from build123d import *

# Parameters (mm, degrees)
SKETCH_R   = 14.3256
SKETCH_R_2 = 38.1
PAD_DEPTH  = 10.000005


with BuildPart() as part:
    # Sketch → Pad (new body)
    with BuildSketch(Plane.XY):
        with BuildLine():
            Line((0, 304.8), (0, 0))
            Line((0, 0), (-203.3016, 0))
            Line((-203.3016, 0), (-203.3016, 304.8))
            ThreePointArc((0, 304.8), (-101.6508, 400.298945), (-203.3016, 304.8))
        make_face()
        with Locations((-152.4, 50.9016)):
            Circle(SKETCH_R, mode=Mode.SUBTRACT)
        with Locations((-50.9016, 50.9016)):
            Circle(SKETCH_R, mode=Mode.SUBTRACT)
        with Locations((-152.4, 152.4)):
            Circle(SKETCH_R, mode=Mode.SUBTRACT)
        with Locations((-50.8, 152.4)):
            Circle(SKETCH_R, mode=Mode.SUBTRACT)
        with Locations((-152.4, 254)):
            Circle(SKETCH_R, mode=Mode.SUBTRACT)
        with Locations((-50.8, 254)):
            Circle(SKETCH_R, mode=Mode.SUBTRACT)
        with Locations((-101.6, 304.8)):
            Circle(SKETCH_R_2, mode=Mode.SUBTRACT)
    extrude(amount=PAD_DEPTH)


solid = part.part
Geometry: final body of the model. Coordinates: model frame, mm. Give positions to 0.01 mm unless a question says otherwise; leave off trailing zeros. Loops run counter-clockwise (first coordinate to the right, second up) from the corner with the lowest first, then second, coordinate; pieces in that order, holes last. Notation, with made-up numbers: (4, 45) - (14, 45) arc R5 cw to (14, 51) - close; hole circle Ø6 at (-25, 34). An arc over 180 degrees is marked (long way). One line per question, with ' | ' between items. Start each with the question number.
(1) Section query C-C on z = 1.75. Return loops of the section in (x, y).
(2) Ray query, line 1 (X direction, y = 253, z = 6); line 2 (Y direction, x = -50.8, z = 3.25); line 3 (Y direction, x = -57.5, z = 4). Return the intervals inside material, ascending. Write a range as from..to.
(3) Pull-direction query (X, two-part tool) for faces 1 (the cylindrical face through (-53.906, 240.015, 4.93)), 2 (the flat face through (-203.302, 150, 5)), 3 (the flat face through (-100, 0, 5)), 4 (the cylindrical face through (-84.02, 271, 4.93)); classes: released by +X, released by -X, zero draft, split by the parting line, or undercut.
(4) Section query A-A on y = 254. Return loops of the section in (x, z), then the cut area to 3 significant figures.
(5) Section query B-B on x = -132. Return loops of the section in (y, z), then the cut area to 3 significant figures.
(6) Contact query for a flat-ended pin moving along its axis: pin 1 (4 mm diameter, centred on x = -39, z = 8.5, fed in from +Y). Output: stop coordinate, or through.
(7) Section query D-D on x = -162. Return loops of the section in (y, z).
The answers:
1) outline: (-203.3, 0) - (0, 0) - (0, 304.8) arc R101.85 ccw to (-203.3, 304.8) - close; hole circle Ø28.65 at (-152.4, 50.9); hole circle Ø28.65 at (-152.4, 152.4); hole circle Ø28.65 at (-152.4, 254); hole circle Ø76.2 at (-101.6, 304.8); hole circle Ø28.65 at (-50.9, 50.9); hole circle Ø28.65 at (-50.8, 152.4); hole circle Ø28.65 at (-50.8, 254)
2) line 1: -203.3..-166.69, -138.11..-65.09, -36.51..0 | line 2: 0..36.58, 65.23..138.07, 166.73..239.67, 268.33..386.7 | line 3: 0..38.19, 63.62..139.74, 165.06..241.34, 266.66..390.23
3) face 1: undercut | face 2: released by -X | face 3: zero draft | face 4: undercut
4) outline: (-203.3, 0) - (-166.73, 0) - (-166.73, 10) - (-203.3, 10) - close; (-138.07, 0) - (-65.13, 0) - (-65.13, 10) - (-138.07, 10) - close; (-36.47, 0) - (0, 0) - (0, 10) - (-36.47, 10) - close | area: 1,460 mm2
5) outline: (0, 0) - (281.83, 0) - (281.83, 10) - (0, 10) - close; (327.77, 0) - (395.67, 0) - (395.67, 10) - (327.77, 10) - close | area: 3,500 mm2
6) pin 1: y = 380.27
7) outline: (0, 0) - (40.27, 0) - (40.27, 10) - (0, 10) - close; (61.53, 0) - (141.77, 0) - (141.77, 10) - (61.53, 10) - close; (163.03, 0) - (243.37, 0) - (243.37, 10) - (163.03, 10) - close; (264.63, 0) - (380.49, 0) - (380.49, 10) - (264.63, 10) - close
